```python
from build123d import *

# Parameters (mm, degrees)
F0_W      = 51.35
F0_H      = 63.35
F1_DEPTH  = 3.175
F3_DEPTH  = 30.5
F5_DEPTH  = 3.175
F7_DEPTH  = 3.175
F9_DEPTH  = 45
F11_DEPTH = 3.175


with BuildPart() as f1:
    # F0 (on Top) → F1 (new body)
    with BuildSketch(Plane.XY):
        with Locations((22.5, -28.5)):
            Rectangle(F0_W, F0_H)
        Polygon((0, -57), (0, 0), (22.5, 0), (45, 0), (45, -57), (40, -57), (40, -54.75), (22.5, -54.75), (5, -54.75), (5, -57), align=None, mode=Mode.SUBTRACT)
        Polygon((22.5, 0), (0, 0), (0, -57), (5, -57), (5, -54.75), (22.5, -54.75), align=None)
        Polygon((45, 0), (22.5, 0), (22.5, -54.75), (40, -54.75), (40, -57), (45, -57), align=None)
    extrude(amount=F1_DEPTH)

    # F2 (on face) → F3 (join)
    with BuildSketch(Plane.XY.offset(3.175)):
        Polygon((0, -19.05), (0, 0), (22.5, 0), (45, 0), (45, -19.05), (48.175, -19.05), (48.175, 3.175), (-3.175, 3.175), (-3.175, -19.05), align=None)
    extrude(amount=F3_DEPTH)

    # F4 (on face) → F5 (join, through all)
    with BuildSketch(Plane.YZ.offset(48.175)):
        Polygon((-19.05, 36.85), (-19.05, 33.675), (3.175, 33.675), align=None)
        Polygon((-19.05, 40.057234329), (-19.05, 36.85), (3.175, 33.675), (3.175, 36.882234329), align=None)
    extrude(amount=-F5_DEPTH)

    # F6 (on face) → F7 (join, through all)
    with BuildSketch(Plane(origin=(-3.175, 0, 0), x_dir=(0, -1, 0), z_dir=(-1, 0, 0))):
        Polygon((-3.175, 33.675), (19.05, 36.85), (19.05, 40.057234329), (-3.175, 36.882234329), align=None)
        Polygon((-3.175, 33.675), (19.05, 33.675), (19.05, 36.85), align=None)
    extrude(amount=-F7_DEPTH)

    # F8 (on face) → F9 (join, through all)
    with BuildSketch(Plane.YZ):
        Polygon((-19.05, 40.057234329), (-19.05, 36.85), (0, 34.1285714286), (0, 33.675), (3.175, 33.675), (3.175, 36.882234329), align=None)
    extrude(amount=F9_DEPTH)

    # F10 (on face) → F11 (join)
    with BuildSketch(Plane.XY.offset(3.175)):
        Polygon((40, -54.75), (22.5, -54.75), (5, -54.75), (5, -57), (0, -57), (0, -60.175), (45, -60.175), (45, -57), (40, -57), align=None)
    extrude(amount=F11_DEPTH)


solid = f1.part
```
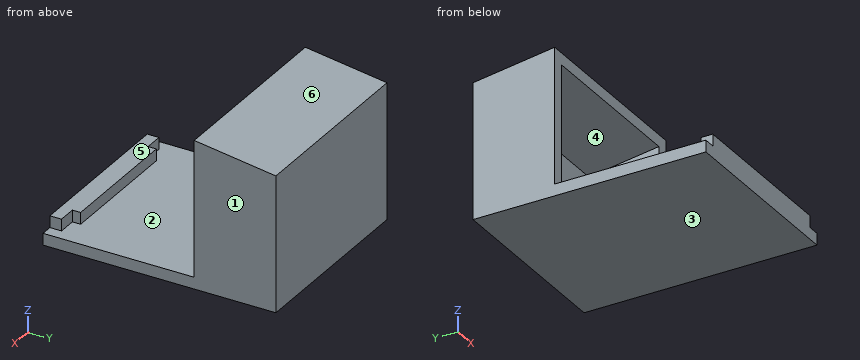
Could you check a few things on this model? Use its own coordinates, in mm. Face numbers are marked on the shaded views. A direction names the side the tool comes from. Coordinates: 2 decimals unless noted, no trailing zeros. Order: outer loops, then holes, each group sorted by start corner. A loop starts at its lowest first (then second) coordinate and runs counter-clockwise, first axis right, second up. Notation, with made-up numbers: M 63,69 L 90,69 A32 cw 90,96 Z; hole C 21,15 d7. An arc over 180 degrees is marked long. Use one line per item in the form item = value. Start each with the question number.
1. For pin 1 (2.5 mm diameter, centred on y = -55.5, z = 4.5, fed in from +X); pin 2 (2.5 mm diameter, centred on y = -58.5, z = 4.5, fed in from -X); pin 3 (1 mm diameter, centred on y = -58, z = 4, fed in from +X), each with a flat end and sliding along its axis, tell me the tip position at first contact or that it passes through.
2. Suppose I cut it at C-C on z = 11. Write out the boundary of the cut face in (x, y) (3 decimals).
3. On a 3-axis mill with a long thin cutter (end or side, diameter ignored), from which of +Z, -Z, +X, -X, +Y, -Y can I reach the whole of each face in a straight line? I mean the marked faces 4, 5 and 6. Say none if no direction works.
4. Suppose I cut it at A-A on z = 5.5. Write out the boundary of the cut face in (x, y) (3 decimals), then the cut area to 3 significant figures.
5. Suppose I cut it at B-B on y = -12. Write out the boundary of the cut face in (x, z) (3 decimals), then the cut area to 3 significant figures.
6. Suppose I cut it at D-D on x = 21. Write out the boundary of the cut face in (y, z) (3 decimals).
7. We'd pull the mould along X, two halves only. Please class the marked faces 1, 2 and 3: +X half, -X half, draft (parallel to the pull), parting line (faces both ways), or undercut.
8. Please list where these lines run through material, in increasing order: line 1 (X direction, y = -18.5, z = 27) (3 decimals); line 2 (Z direction, x = 1, y = -55.5) (3 decimals).
Geometry says:
q1.pin_1 = 40
q1.pin_2 = 0
q1.pin_3 = 45
q2.outline = M -3.175,-19.05 L 0,-19.05 L 0,0 L 45,0 L 45,-19.05 L 48.175,-19.05 L 48.175,3.175 L -3.175,3.175 Z
q3.face_4 = -Y
q3.face_5 = +Z, +X, -X, -Y
q3.face_6 = +Z, +X, -X, +Y
q4.outline = M -3.175,-19.05 L 0,-19.05 L 0,0 L 45,0 L 45,-19.05 L 48.175,-19.05 L 48.175,3.175 L -3.175,3.175 Z; M 0,-60.175 L 45,-60.175 L 45,-57 L 40,-57 L 40,-54.75 L 5,-54.75 L 5,-57 L 0,-57 Z
q4.area = 506 mm^2
q5.outline = M -3.175,0 L 48.175,0 L 48.175,39.05 L -3.175,39.05 Z; hole M 0,3.175 L 45,3.175 L 45,35.843 L 0,35.843 Z
q5.area = 535 mm^2
q6.outline = M -60.175,0 L 3.175,0 L 3.175,36.882 L -19.05,40.057 L -19.05,36.85 L 0,34.129 L 0,3.175 L -54.75,3.175 L -54.75,6.35 L -60.175,6.35 Z
q7.face_1 = +X half
q7.face_2 = undercut
q7.face_3 = draft
q8.line_1 = -3.175 to 0, 45 to 48.175
q8.line_2 = 0 to 3.175
